Geometry check sheet. Reference: the model listing, model coordinates, mm. Face numbers are marked on the shaded views. A direction names the side the tool comes from. Coordinates: 2 decimals unless noted, no trailing zeros. Loops run counter-clockwise (first coordinate to the right, second up) from the corner with the lowest first, then second, coordinate; pieces in that order, holes last. Notation, with made-up numbers: (74.5, 59) - (95.5, 59) arc R19 cw to (95.5, 94) - close; hole circle Ø2 at (42, 6.5). An arc over 180 degrees is marked (long way). One line per item, written item: value.
from build123d import *

# Parameters (mm, degrees)
BOSS_EXTRUDE1_DEPTH = 5
FILLET1_R           = 6
CHAMFER1_SIZE       = 3
CHAMFER1_SIZE2      = 5.196152423
CHAMFER2_SIZE       = 3
CHAMFER2_SIZE2      = 5.196152423
CUT_EXTRUDE1_REACH  = 165.86
SKETCH4_R           = 1.6
CUT_EXTRUDE2_REACH  = 174.772
SKETCH5_W           = 85
SKETCH5_H           = 1
FILLET3_R           = 5


# Some blends are built 0.0001 mm under size
with BuildPart() as part:
    # Sketch2 → Boss-Extrude1 (new body)
    with BuildSketch(Plane(origin=(0, 0, 0), x_dir=(1, 0, 0), z_dir=(0, 1, 0))):
        Polygon((15, 0), (-15, 0), (-15, -70), (-27, -70), (-27, -2), (-35, -2), (-35, -22), (-30, -22), (-30, -160), (30, -160), (30, -22), (35, -22), (35, -2), (27, -2), (27, -70), (15, -70), align=None)
    extrude(amount=BOSS_EXTRUDE1_DEPTH)

    # Fillet1
    fillet1_edges = [part.edges().sort_by_distance(p)[0] for p in [
        (-27, 2.5, 70),
        (-15, 2.5, 70),
        (15, 2.5, 70),
        (27, 2.5, 70),
        (-35, 2.5, 2),
        (35, 2.5, 2),
    ]]
    fillet(fillet1_edges, radius=FILLET1_R - 0.0001)  # a hair under: the kernel refuses the full size

    # Chamfer1
    chamfer1_edges = [part.edges().sort_by_distance(p)[0] for p in [
        (-30, 2.5, 22),
    ]]
    chamfer1_side = [part.faces().sort_by_distance(p)[0] for p in [
        (-32.5, 2.5, 22),
    ]]
    chamfer(chamfer1_edges, length=CHAMFER1_SIZE, length2=CHAMFER1_SIZE2, reference=chamfer1_side[0])

    # Chamfer2
    chamfer2_edges = [part.edges().sort_by_distance(p)[0] for p in [
        (30, 2.5, 22),
    ]]
    chamfer2_side = [part.faces().sort_by_distance(p)[0] for p in [
        (32.5, 2.5, 22),
    ]]
    chamfer(chamfer2_edges, length=CHAMFER2_SIZE, length2=CHAMFER2_SIZE2, reference=chamfer2_side[0])

    # Sketch4 → Cut-Extrude1 (cut, up to next)
    with BuildSketch(Plane(origin=(0, 5, 0), x_dir=(1, 0, 0), z_dir=(0, 1, 0)), mode=Mode.PRIVATE) as cut_extrude1_sk1:
        with Locations(Location((-20, -152, 0), (0, 0, 270))):
            Circle(SKETCH4_R)
    cut_extrude1_tool1 = extrude(cut_extrude1_sk1.sketch, amount=-CUT_EXTRUDE1_REACH, mode=Mode.PRIVATE) & part.part
    # Sketch4 → Cut-Extrude1 (cut, up to next)
    with BuildSketch(Plane(origin=(0, 5, 0), x_dir=(1, 0, 0), z_dir=(0, 1, 0)), mode=Mode.PRIVATE) as cut_extrude1_sk2:
        with Locations(Location((20, -152, 0), (0, 0, 270))):
            Circle(SKETCH4_R)
    cut_extrude1_tool2 = extrude(cut_extrude1_sk2.sketch, amount=-CUT_EXTRUDE1_REACH, mode=Mode.PRIVATE) & part.part
    # Sketch4 → Cut-Extrude1 (cut, up to next)
    with BuildSketch(Plane(origin=(0, 5, 0), x_dir=(1, 0, 0), z_dir=(0, 1, 0)), mode=Mode.PRIVATE) as cut_extrude1_sk3:
        with Locations(Location((-20, -127, 0), (0, 0, 270))):
            Circle(SKETCH4_R)
    cut_extrude1_tool3 = extrude(cut_extrude1_sk3.sketch, amount=-CUT_EXTRUDE1_REACH, mode=Mode.PRIVATE) & part.part
    # Sketch4 → Cut-Extrude1 (cut, up to next)
    with BuildSketch(Plane(origin=(0, 5, 0), x_dir=(1, 0, 0), z_dir=(0, 1, 0)), mode=Mode.PRIVATE) as cut_extrude1_sk4:
        with Locations(Location((20, -127, 0), (0, 0, 270))):
            Circle(SKETCH4_R)
    cut_extrude1_tool4 = extrude(cut_extrude1_sk4.sketch, amount=-CUT_EXTRUDE1_REACH, mode=Mode.PRIVATE) & part.part
    add(cut_extrude1_tool1.solids().sort_by_distance((-20, 5, 152))[0], mode=Mode.SUBTRACT)
    add(cut_extrude1_tool2.solids().sort_by_distance((20, 5, 152))[0], mode=Mode.SUBTRACT)
    add(cut_extrude1_tool3.solids().sort_by_distance((-20, 5, 127))[0], mode=Mode.SUBTRACT)
    add(cut_extrude1_tool4.solids().sort_by_distance((20, 5, 127))[0], mode=Mode.SUBTRACT)

    # Sketch5 → Cut-Extrude2 (cut, up to next)
    with BuildSketch(Plane.ZY.offset(30), mode=Mode.PRIVATE) as cut_extrude2_sk1:
        with Locations((117.5, 0.5)):
            Rectangle(SKETCH5_W, SKETCH5_H)
    cut_extrude2_tool1 = extrude(cut_extrude2_sk1.sketch, amount=-CUT_EXTRUDE2_REACH, mode=Mode.PRIVATE) & part.part
    add(cut_extrude2_tool1.solids().sort_by_distance((-30, 0.5, 117.5))[0], mode=Mode.SUBTRACT)

    # Fillet3
    # the kernel refuses this fillet: 5 mm, written as the material it adds along each edge
    with BuildSketch(Plane(origin=(-30, 1, 75), x_dir=(0, -1, 0), z_dir=(1, 0, 0))) as fillet3_piece_1:
        with BuildLine():
            CenterArc((5, -3), FILLET3_R, 143.130102354, 36.869897646)
            Line((0, -3), (-0.1, -3))
            Line((-0.1, -3), (-0.1, 0))
            Line((-0.1, 0), (0, 0.1))
            ThreePointArc((0, 0.1), (0.5, 0.1), (0.92, 0.06))
            Line((0.92, 0.06), (1, 0))
        make_face()
    extrude(amount=60)


solid = part.part
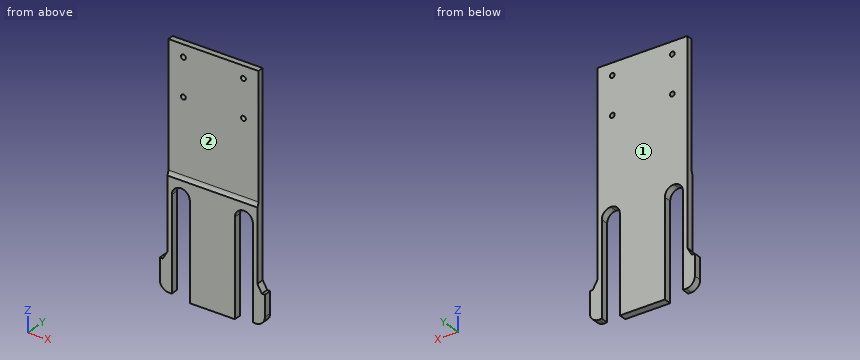
(1) Access from +Z, -Z, +X, -X, +Y, -Y to the whole of each face (thin tool, end or side, straight path). Record for the marked faces 1 and 2.
Reply:
face 1: +Z, -Z, +X, -X, +Y
face 2: +Z, +X, -X, -Y
(2) Cross-section at D-D on z = 24. Record the cut outline in (x, y).
Reply:
outline: (-31.85, 0) - (-27, 0) - (-27, 5) - (-31.85, 5) - close; (-15, 0) - (15, 0) - (15, 5) - (-15, 5) - close; (27, 0) - (31.85, 0) - (31.85, 5) - (27, 5) - close
(3) Cross-section at C-C on x = 0.5. Record the cut outline in (y, z).
Reply:
outline: (0, 0) - (5, 0) - (5, 160) - (1, 160) - (1, 78) arc R5 cw to (0, 75) - close
(4) Material ranges on probe 1 along X at (y, z) = (2.15, 127); probe 2 along Z at (x, y) = (-28.5, 4.25); probe 3 along Z at (x, y) = (-20.5, 1.1), recorded low to high. Write a range as from..to.
Reply:
probe 1: -30..-21.6, -18.4..18.4, 21.6..30
probe 2: 2..160
probe 3: 69.98..125.48, 128.52..150.48, 153.52..160
(5) Cross-section at B-B on y = 3.85. State how many separate pieces and enclosed holes the cut face has, and give its area (3 significant figures).
Reply:
separate pieces: 1
enclosed holes: 4
area: 8,110 mm2
(6) Cross-section at A-A on z = 152. Record the cut outline in (x, y), and give its area (3 significant figures).
Reply:
outline: (-30, 1) - (-21.6, 1) - (-21.6, 5) - (-30, 5) - close; (-18.4, 1) - (18.4, 1) - (18.4, 5) - (-18.4, 5) - close; (21.6, 1) - (30, 1) - (30, 5) - (21.6, 5) - close
area: 214 mm2
(7) Go/stop test with flat-tipped pins: pin 1 Ø3.5 at (x, z) = (20, 127) entering from -Y; pin 2 Ø1.6 at (x, y) = (-34.5, 2.5) entering from +Z; pin 3 Ø2 at (y, z) = (3, 40) entering from -X. Record where each tip stops, or that it passes through.
Reply:
pin 1: y = 1
pin 2: z = 22
pin 3: x = -30
